Geometry: final body of the model. Coordinates: model frame, mm. A direction names the side the tool comes from. Coordinates: 2 decimals unless noted, no trailing zeros. Loops run counter-clockwise (first coordinate to the right, second up) from the corner with the lowest first, then second, coordinate; pieces in that order, holes last. Notation, with made-up numbers: (-40, -23.75) -> (-26, -23.75) arc R33 ccw to (-26, 5.25) -> close; hole circle Ø2 at (26, 46.5). An arc over 180 degrees is marked (long way). One line per item, written item: value. Start each with the question number.
Item 1: Contact query for flat-ended pins moving along their axis: pin 1 Ø3.5 at (x, y) = (12.895, 20.865) entering from +Z; pin 2 Ø5.5 at (x, y) = (12.895, 20.865) entering from +Z. Output: stop coordinate, or through.
Item 2: Section query A-A on x = 6.5. Return loops of the section in (y, z).
Item 3: Section query B-B on y = 20.25. Return loops of the section in (x, z), then the cut area to 3 significant figures.
Item 4: Set-up query: faces 4 (the cylindrical face through (6.309, 2.263, 4.754)), 5 (the flat face through (9, 13, 0)). Return all of +Z, -Z, +X, -X, +Y, -Y with unobstructed straight access to the full face (end or side cutting, diameter ignored); none if empty.
Item 5: Ray query, probe 1 along X at (y, z) = (5, 1.35); probe 2 along Y at (x, z) = (2.75, 4.2); probe 3 along Y at (x, z) = (3.25, 2.55). Return the intervals inside material, ascending. Write a range as from..to.
Item 6: Mould query, pull axis X, two halves, no side actions, for faces 1 (the flat face through (9, 13, 5)), 2 (the cylindrical face through (12.58, 23.27, 2.28)), 3 (the flat face through (17.82, 13, 2)). Classes: +X half, -X half, draft (parallel to the pull), parting line (faces both ways), or undercut.
Item 7: Section query C-C on z = 3.1. Return loops of the section in (x, y) (3 decimals).
from build123d import *

# Parameters (mm, degrees)
SKETCH1_W           = 17.82
SKETCH1_H           = 25.79
BOSS_EXTRUDE2_DEPTH = 5
SKETCH2_R           = 2.425
CUT_EXTRUDE1_DEPTH  = 15
SKETCH3_R           = 3
CUT_EXTRUDE2_DEPTH  = 0.5


with BuildPart() as part:
    # Sketch1 → Boss-Extrude2 (new body)
    with BuildSketch(Plane.XY):
        with Locations((8.91, 12.895)):
            Rectangle(SKETCH1_W, SKETCH1_H)
    extrude(amount=BOSS_EXTRUDE2_DEPTH)

    # Sketch2 → Cut-Extrude1 (cut)
    with BuildSketch(Plane.XY.offset(5)):
        with Locations((4.925, 4.925)):
            Circle(SKETCH2_R)
        with Locations((12.895, 20.865)):
            Circle(SKETCH2_R)
    extrude(amount=-CUT_EXTRUDE1_DEPTH, mode=Mode.SUBTRACT)

    # Sketch3 → Cut-Extrude2 (cut)
    with BuildSketch(Plane.XY.offset(5)):
        with Locations((4.925, 4.925)):
            Circle(SKETCH3_R)
        with Locations((12.895, 20.865)):
            Circle(SKETCH3_R)
    extrude(amount=-CUT_EXTRUDE2_DEPTH, mode=Mode.SUBTRACT)


solid = part.part
Reply:
1. pin 1: passes through
1. pin 2: stops at z = 4.5
2. outline: (0, 0) -> (3.08, 0) -> (3.08, 4.5) -> (2.37, 4.5) -> (2.37, 5) -> (0, 5) -> close; (6.77, 0) -> (25.79, 0) -> (25.79, 5) -> (7.48, 5) -> (7.48, 4.5) -> (6.77, 4.5) -> close
3. outline: (0, 0) -> (10.55, 0) -> (10.55, 4.5) -> (9.96, 4.5) -> (9.96, 5) -> (0, 5) -> close; (15.24, 0) -> (17.82, 0) -> (17.82, 5) -> (15.83, 5) -> (15.83, 4.5) -> (15.24, 4.5) -> close
3. area: 65.1 mm²
4. face 4: +Z
4. face 5: -Z, +X, -X, +Y, -Y
5. probe 1: x = 0..2.5, 7.35..17.82
5. probe 2: y = 0..3.85, 6..25.79
5. probe 3: y = 0..3.17, 6.68..25.79
6. face 1: draft
6. face 2: undercut
6. face 3: +X half
7. outline: (0, 0) -> (17.82, 0) -> (17.82, 25.79) -> (0, 25.79) -> close; hole circle Ø4.85 at (4.925, 4.925); hole circle Ø4.85 at (12.895, 20.865)
